Check sheet for the modelled part. Datum: model origin and axes. Units: mm. A direction names the side the tool comes from. Give positions to 0.01 mm unless a question says otherwise; leave off trailing zeros. Order: outer loops, then holes, each group sorted by start corner. A loop starts at its lowest first (then second) coordinate and runs counter-clockwise, first axis right, second up. Notation, with made-up numbers: (79, 51.25) - (98, 51.25) arc R22 ccw to (98, 58.25) - close; hole circle Ø10 at (71.5, 14.5). An arc over 180 degrees is marked (long way). Answer in a Markdown table with one row per item.
from build123d import *

# Parameters (mm, degrees)
IZIM1_R                     = 1.5
IZIM1_R_2                   = 1.275
Y_KSEKLIK_EKSTR_ZYON1_DEPTH = 8
IZIM2_R                     = 4
KES_EKSTR_ZYON1_DEPTH       = 5
IZIM3_R                     = 3.5
KES_EKSTR_ZYON2_DEPTH       = 5
IZIM5_W                     = 11.833700998
IZIM5_H                     = 5.687133077
Y_KSEKLIK_EKSTR_ZYON2_DEPTH = 55
IZIM6_R                     = 1.5
KES_EKSTR_ZYON3_DEPTH       = 70
Y_KSEKLIK_EKSTR_ZYON3_DEPTH = 10
KES_EKSTR_ZYON4_START       = -10
IZIM8_R                     = 1.5
KES_EKSTR_ZYON4_DEPTH       = 10
IZIM9_W                     = 97.77314617
IZIM9_H                     = 81.30293778
KES_EKSTR_ZYON5_DEPTH       = 94.5
IZIM10_R                    = 3
IZIM10_R_2                  = 1.35
Y_KSEKLIK_EKSTR_ZYON4_DEPTH = 5
IZIM12_R                    = 1.35
KES_EKSTR_ZYON6_DEPTH       = 11.5


with BuildPart() as part:
    # Çizim1 → Yükseklik-Ekstrüzyon1 (new body)
    with BuildSketch(Plane.XY):
        with BuildLine():
            Line((-26.942326891, 14.769848309), (-15.036455376, 14.769848309))
            ThreePointArc((-15.036455376, 14.769848309), (-11.50092147, 13.305382214), (-10.036455376, 9.769848309))
            Line((-10.036455376, 9.769848309), (-10.036455376, -8.006371062))
            ThreePointArc((-10.036455376, -8.006371062), (-11.50092147, -11.541904968), (-15.036455376, -13.006371062))
            Line((-15.036455376, -13.006371062), (-26.942326891, -13.006371062))
            ThreePointArc((-26.942326891, -13.006371062), (-30.477860797, -14.470837156), (-31.942326891, -18.006371062))
            Line((-31.942326891, -18.006371062), (-31.942326891, -21.470074229))
            ThreePointArc((-31.942326891, -21.470074229), (-31.6091093, -24.030019123), (-30.63166332, -26.419360282))
            Line((-30.63166332, -26.419360282), (-25.398075072, -35.607838889))
            ThreePointArc((-25.398075072, -35.607838889), (-21.734031643, -39.304154624), (-16.708738643, -40.658552836))
            Line((-16.708738643, -40.658552836), (16.824084861, -40.658552836))
            ThreePointArc((16.824084861, -40.658552836), (21.849377861, -39.304154624), (25.513421289, -35.607838889))
            Line((25.513421289, -35.607838889), (30.747009537, -26.419360282))
            ThreePointArc((30.747009537, -26.419360282), (31.724455518, -24.030019123), (32.057673109, -21.470074229))
            Line((32.057673109, -21.470074229), (32.057673109, -18.006371062))
            ThreePointArc((32.057673109, -18.006371062), (30.593207015, -14.470837156), (27.057673109, -13.006371062))
            Line((27.057673109, -13.006371062), (15.151801594, -13.006371062))
            ThreePointArc((15.151801594, -13.006371062), (11.616267688, -11.541904968), (10.151801594, -8.006371062))
            Line((10.151801594, -8.006371062), (10.151801594, 9.769848309))
            ThreePointArc((10.151801594, 9.769848309), (11.616267688, 13.305382214), (15.151801594, 14.769848309))
            Line((15.151801594, 14.769848309), (27.057673109, 14.769848309))
            ThreePointArc((27.057673109, 14.769848309), (30.593207015, 16.234314403), (32.057673109, 19.769848309))
            Line((32.057673109, 19.769848309), (32.057673109, 23.233551476))
            ThreePointArc((32.057673109, 23.233551476), (31.724455518, 25.793496369), (30.747009537, 28.182837528))
            Line((30.747009537, 28.182837528), (25.513421289, 37.371316135))
            ThreePointArc((25.513421289, 37.371316135), (21.849377861, 41.06763187), (16.824084861, 42.422030083))
            Line((16.824084861, 42.422030083), (-16.708738643, 42.422030083))
            ThreePointArc((-16.708738643, 42.422030083), (-21.734031643, 41.06763187), (-25.398075072, 37.371316135))
            Line((-25.398075072, 37.371316135), (-30.63166332, 28.182837528))
            ThreePointArc((-30.63166332, 28.182837528), (-31.6091093, 25.793496369), (-31.942326891, 23.233551476))
            Line((-31.942326891, 23.233551476), (-31.942326891, 19.769848309))
            ThreePointArc((-31.942326891, 19.769848309), (-30.477860797, 16.234314403), (-26.942326891, 14.769848309))
        make_face()
        with Locations((20.284256069, 32.422030083)):
            Circle(IZIM1_R, mode=Mode.SUBTRACT)
        with Locations((-20.168909852, 32.422030083)):
            Circle(IZIM1_R, mode=Mode.SUBTRACT)
        with Locations((-20.168909852, -30.658552836)):
            Circle(IZIM1_R, mode=Mode.SUBTRACT)
        with Locations((20.284256069, -30.658552836)):
            Circle(IZIM1_R, mode=Mode.SUBTRACT)
        with Locations((22.057673109, -21.118261377)):
            Circle(IZIM1_R_2, mode=Mode.SUBTRACT)
        with Locations((-21.942326891, -21.118261377)):
            Circle(IZIM1_R_2, mode=Mode.SUBTRACT)
        with Locations((22.057673109, 22.881738623)):
            Circle(IZIM1_R_2, mode=Mode.SUBTRACT)
        with Locations((-21.942326891, 22.881738623)):
            Circle(IZIM1_R_2, mode=Mode.SUBTRACT)
        with Locations((0.057673109, 32.422030083)):
            Circle(IZIM1_R, mode=Mode.SUBTRACT)
        with Locations(Location((0.057673109, -30.658552836, 0), (0, 0, 180))):
            Circle(IZIM1_R, mode=Mode.SUBTRACT)
    extrude(amount=Y_KSEKLIK_EKSTR_ZYON1_DEPTH)

    # Çizim2 → Kes-Ekstrüzyon1 (cut)
    with BuildSketch(Plane(origin=(0, 0, 0), x_dir=(-1, 0, 0), z_dir=(0, 0, -1))):
        with Locations((-22.057673109, 22.881738623)):
            Circle(IZIM2_R)
        with Locations((21.942326891, 22.881738623)):
            Circle(IZIM2_R)
        with Locations((-22.057673109, -21.118261377)):
            Circle(IZIM2_R)
        with Locations((21.942326891, -21.118261377)):
            Circle(IZIM2_R)
        with Locations((-0.057673109, 32.422030083)):
            Circle(IZIM2_R)
        with Locations((-0.057673109, -30.658552836)):
            Circle(IZIM2_R)
    extrude(amount=-KES_EKSTR_ZYON1_DEPTH, mode=Mode.SUBTRACT)

    # Çizim3 → Kes-Ekstrüzyon2 (cut)
    with BuildSketch(Plane.XY.offset(8)):
        with Locations((-20.168909852, 32.422030083)):
            Circle(IZIM3_R)
        with Locations((20.284256069, 32.422030083)):
            Circle(IZIM3_R)
        with Locations((20.284256069, -30.658552836)):
            Circle(IZIM3_R)
        with Locations((-20.168909852, -30.658552836)):
            Circle(IZIM3_R)
    extrude(amount=-KES_EKSTR_ZYON2_DEPTH, mode=Mode.SUBTRACT)

    # Çizim5 → Yükseklik-Ekstrüzyon2 (add)
    with BuildSketch(Plane.XY.offset(8)):
        with Locations((0.057673109, 32.422030083)):
            Rectangle(IZIM5_W, IZIM5_H)
        with Locations((0.057673109, -30.658552837)):
            Rectangle(IZIM5_W, IZIM5_H)
    extrude(amount=Y_KSEKLIK_EKSTR_ZYON2_DEPTH)

    # Çizim6 → Kes-Ekstrüzyon3 (cut)
    with BuildSketch(Plane(origin=(0, 0, 8), x_dir=(-1, 0, 0), z_dir=(0, 0, -1))):
        with Locations((-0.057673109, -30.658552836)):
            Circle(IZIM6_R)
        with Locations((-0.057673109, 32.422030083)):
            Circle(IZIM6_R)
    extrude(amount=-KES_EKSTR_ZYON3_DEPTH, mode=Mode.SUBTRACT)

    # Çizim7 → Yükseklik-Ekstrüzyon3 (add)
    with BuildSketch(Plane.XY.offset(63)):
        with BuildLine():
            Line((-31.942326891, 23.233551476), (-31.942326891, 19.769848309))
            ThreePointArc((-31.942326891, 19.769848309), (-30.477860797, 16.234314403), (-26.942326891, 14.769848309))
            Line((-26.942326891, 14.769848309), (-15.036455376, 14.769848309))
            ThreePointArc((-15.036455376, 14.769848309), (-11.50092147, 13.305382214), (-10.036455376, 9.769848309))
            Line((-10.036455376, 9.769848309), (-10.036455376, -8.006371062))
            ThreePointArc((-10.036455376, -8.006371062), (-11.50092147, -11.541904968), (-15.036455376, -13.006371062))
            Line((-15.036455376, -13.006371062), (-26.942326891, -13.006371062))
            ThreePointArc((-26.942326891, -13.006371062), (-30.477860797, -14.470837156), (-31.942326891, -18.006371062))
            Line((-31.942326891, -18.006371062), (-31.942326891, -21.470074229))
            ThreePointArc((-31.942326891, -21.470074229), (-31.6091093, -24.030019123), (-30.63166332, -26.419360282))
            Line((-30.63166332, -26.419360282), (-25.398075072, -35.607838889))
            ThreePointArc((-25.398075072, -35.607838889), (-21.734031643, -39.304154624), (-16.708738643, -40.658552836))
            Line((-16.708738643, -40.658552836), (16.824084861, -40.658552836))
            ThreePointArc((16.824084861, -40.658552836), (21.849377861, -39.304154624), (25.513421289, -35.607838889))
            Line((25.513421289, -35.607838889), (30.747009537, -26.419360282))
            ThreePointArc((30.747009537, -26.419360282), (31.724455518, -24.030019123), (32.057673109, -21.470074229))
            Line((32.057673109, -21.470074229), (32.057673109, -18.006371062))
            ThreePointArc((32.057673109, -18.006371062), (30.593207015, -14.470837156), (27.057673109, -13.006371062))
            Line((27.057673109, -13.006371062), (15.151801594, -13.006371062))
            ThreePointArc((15.151801594, -13.006371062), (11.616267688, -11.541904968), (10.151801594, -8.006371062))
            Line((10.151801594, -8.006371062), (10.151801594, 9.769848309))
            ThreePointArc((10.151801594, 9.769848309), (11.616267688, 13.305382214), (15.151801594, 14.769848309))
            Line((15.151801594, 14.769848309), (27.057673109, 14.769848309))
            ThreePointArc((27.057673109, 14.769848309), (30.593207015, 16.234314403), (32.057673109, 19.769848309))
            Line((32.057673109, 19.769848309), (32.057673109, 23.233551476))
            ThreePointArc((32.057673109, 23.233551476), (31.724455518, 25.793496369), (30.747009537, 28.182837528))
            Line((30.747009537, 28.182837528), (25.513421289, 37.371316135))
            ThreePointArc((25.513421289, 37.371316135), (21.849377861, 41.06763187), (16.824084861, 42.422030083))
            Line((16.824084861, 42.422030083), (-16.708738643, 42.422030083))
            ThreePointArc((-16.708738643, 42.422030083), (-21.734031643, 41.06763187), (-25.398075072, 37.371316135))
            Line((-25.398075072, 37.371316135), (-30.63166332, 28.182837528))
            ThreePointArc((-30.63166332, 28.182837528), (-31.6091093, 25.793496369), (-31.942326891, 23.233551476))
        make_face()
    extrude(amount=Y_KSEKLIK_EKSTR_ZYON3_DEPTH)

    # Çizim8 → Kes-Ekstrüzyon4 (cut)
    with BuildSketch(Plane.XY.offset(73).offset(KES_EKSTR_ZYON4_START)):
        with Locations(Location((0.057673109, -30.658552836, 0), (0, 0, 180))):
            Circle(IZIM8_R)
        with Locations(Location((0.057673109, 32.422030083, 0), (0, 0, 180))):
            Circle(IZIM8_R)
    extrude(amount=KES_EKSTR_ZYON4_DEPTH, mode=Mode.SUBTRACT)

    # Çizim9 → Kes-Ekstrüzyon5 (cut, symmetric)
    with BuildSketch(Plane(origin=(0, 35.265596621, 0), x_dir=(1, 0, 0), z_dir=(0, 1, 0))):
        with Locations((-4.059878989, -28.264895805)):
            Rectangle(IZIM9_W, IZIM9_H)
    extrude(amount=KES_EKSTR_ZYON5_DEPTH, both=True, mode=Mode.SUBTRACT)

    # Çizim10 → Yükseklik-Ekstrüzyon4 (add)
    # profile 1 of 4: a face of its own
    with BuildSketch(Plane(origin=(0, 0, 68.916364695), x_dir=(-1, 0, 0), z_dir=(0, 0, -1))):
        with Locations(Location((24.673182088, -28.763886305, 0), (0, 0, 180))):
            Circle(IZIM10_R)
        with Locations((24.673182088, -28.763886305)):
            Circle(IZIM10_R_2, mode=Mode.SUBTRACT)
    # profile 2 of 4: a face of its own
    with BuildSketch(Plane(origin=(0, 0, 68.916364695), x_dir=(-1, 0, 0), z_dir=(0, 0, -1))):
        with Locations(Location((-24.326817912, -28.763886305, 0), (0, 0, 180))):
            Circle(IZIM10_R)
        with Locations((-24.326817912, -28.763886305)):
            Circle(IZIM10_R_2, mode=Mode.SUBTRACT)
    # profile 3 of 4: a face of its own
    with BuildSketch(Plane(origin=(0, 0, 68.916364695), x_dir=(-1, 0, 0), z_dir=(0, 0, -1))):
        with Locations(Location((-24.326817912, 29.236113695, 0), (0, 0, 180))):
            Circle(IZIM10_R)
        with Locations((-24.326817912, 29.236113695)):
            Circle(IZIM10_R_2, mode=Mode.SUBTRACT)
    # profile 4 of 4: a face of its own
    with BuildSketch(Plane(origin=(0, 0, 68.916364695), x_dir=(-1, 0, 0), z_dir=(0, 0, -1))):
        with Locations(Location((24.673182088, 29.236113695, 0), (0, 0, 180))):
            Circle(IZIM10_R)
        with Locations((24.673182088, 29.236113695)):
            Circle(IZIM10_R_2, mode=Mode.SUBTRACT)
    extrude(amount=Y_KSEKLIK_EKSTR_ZYON4_DEPTH)

    # Çizim12 → Kes-Ekstrüzyon6 (cut, symmetric)
    with BuildSketch(Plane(origin=(0, 0, 68.916364695), x_dir=(-1, 0, 0), z_dir=(0, 0, -1))):
        with Locations(Location((-24.326817912, -28.763886305, 0), (0, 0, 180))):
            Circle(IZIM12_R)
        with Locations(Location((24.673182088, -28.763886305, 0), (0, 0, 180))):
            Circle(IZIM12_R)
        with Locations(Location((24.673182088, 29.236113695, 0), (0, 0, 180))):
            Circle(IZIM12_R)
        with Locations(Location((-24.326817912, 29.236113695, 0), (0, 0, 180))):
            Circle(IZIM12_R)
    extrude(amount=KES_EKSTR_ZYON6_DEPTH, both=True, mode=Mode.SUBTRACT)


solid = part.part
(1) Mould release check, pull along Y, two halves, no side actions. Record for faces 4 (the flat face through (-31.942, -20, 71)), 5 (the flat face through (-28, 32.8, 70.9)), 6 (the cylindrical face through (0.253, 30.935, 70.93)): pulls with the +Y half, pulls with the -Y half, needs draft (parallel to the pull), parting line crosses it, or undercut.
Geometry says:
| item | result |
|---|---|
| face 4 | needs draft |
| face 5 | pulls with the +Y half |
| face 6 | undercut |
(2) Cross-section at B-B, the plane x = -12.5. Record the cut outline in (y, z).
Geometry says:
| item | result |
|---|---|
| outline | (-40.66, 68.92) - (-12.32, 68.92) - (-12.32, 73) - (-40.66, 73) - close; (14.08, 68.92) - (42.42, 68.92) - (42.42, 73) - (14.08, 73) - close |
(3) Cross-section at A-A, the plane z = 65.25. Record the cut outline in (x, y), then the cut area to 3 significant figures.
Geometry says:
| item | result |
|---|---|
| outline | circle Ø6 at (-24.67, -28.76); circle Ø6 at (-24.67, 29.24); circle Ø6 at (24.33, -28.76); circle Ø6 at (24.33, 29.24); hole circle Ø2.7 at (-24.67, -28.76); hole circle Ø2.7 at (-24.67, 29.24); hole circle Ø2.7 at (24.33, -28.76); hole circle Ø2.7 at (24.33, 29.24) |
| area | 90.2 mm² |
(4) Access from +Z, -Z, +X, -X, +Y, -Y to the whole of each face (thin tool, end or side, straight path). Record for faces 1 (the flat face through (-10.036, 1, 71)), 2 (the cylindrical face through (11.58, 13.27, 70.93)), 3 (the cylindrical face through (-23.29, -26.1, 66.45)).
Geometry says:
| item | result |
|---|---|
| face 1 | +Z, -Z, -X |
| face 2 | +Z, -Z, +X |
| face 3 | -Z |
(5) Gauge pin test, flat ends, axial feed: P1, Ø3.5, axis at x = -24.67, y = -28.76, coming from the -Z side; P2, Ø3.5, axis at x = -23.5, z = 71, coming from the +Y side; P3, Ø3.5, axis at y = 1.5, z = 70.5, coming from the -X side; P4, Ø3.5, axis at x = 23, z = 72, coming from the +Y side. Record the tip position at first contact, or that the pin passes through.
Geometry says:
| item | result |
|---|---|
| P1 | z = 63.92 |
| P2 | y = 41.06 |
| P3 | x = -10.04 |
| P4 | y = 41.39 |
(6) Cross-section at C-C, the plane x = -3.5. Record the cut outline in (y, z), then the cut area to 3 significant figures.
Geometry says:
| item | result |
|---|---|
| outline | (-40.66, 68.92) - (42.42, 68.92) - (42.42, 73) - (-40.66, 73) - close |
| area | 339 mm² |
(7) Thickness scan on L1, parallel to Y at x = 15.5, z = 69.75; L2, parallel to Y at x = 25.5, z = 67; L3, parallel to Z at x = 18, y = 19. Record the ranges inside material, lowest first.
Geometry says:
| item | result |
|---|---|
| L1 | -40.66 to -13.01, 14.77 to 42.42 |
| L2 | -31.52 to -29.43, -28.1 to -26, 26.48 to 28.57, 29.9 to 32 |
| L3 | 68.92 to 73 |
(8) Cross-section at D-D, the plane y = -5.5. Record the cut outline in (x, z), then the cut area to 3 significant figures.
Geometry says:
| item | result |
|---|---|
| outline | (-10.04, 68.92) - (10.15, 68.92) - (10.15, 73) - (-10.04, 73) - close |
| area | 82.4 mm² |
